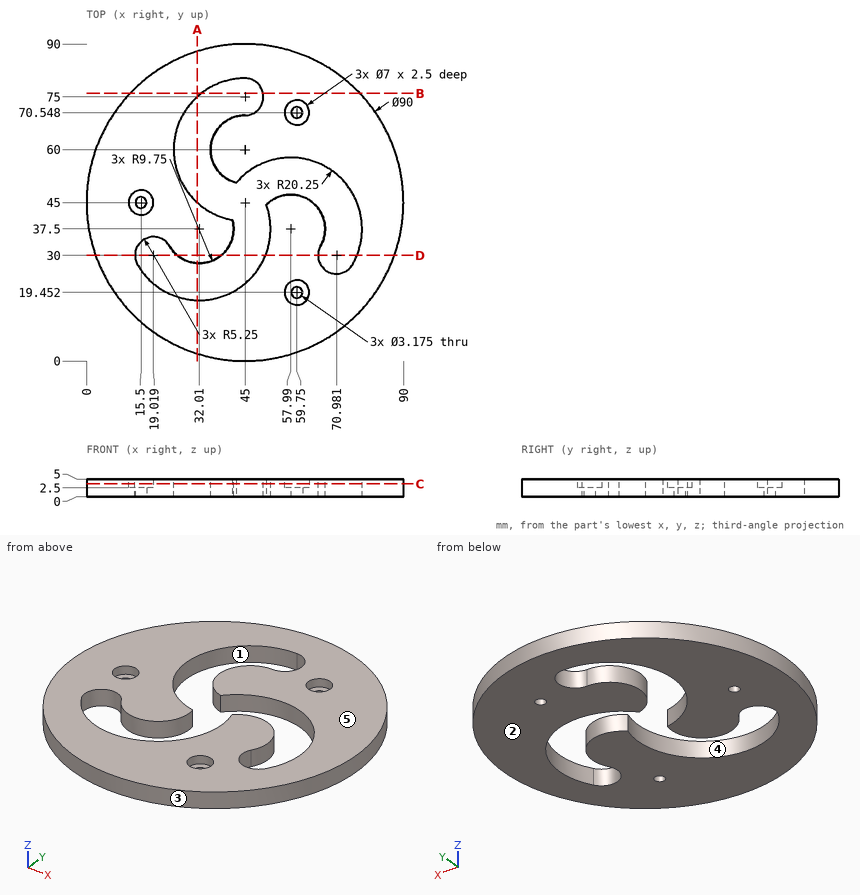
Here's the drawing with two shaded views (mm, measured from the low corner). I have some questions. A direction names the side the tool comes from. Round coordinates to 2 decimals unless told otherwise and drop trailing zeros. Loops run counter-clockwise (first coordinate to the right, second up) from the corner with the lowest first, then second, coordinate; pieces in that order, holes last. Notation, with made-up numbers: M 39,-40 L 74,-40 A33 ccw 74,-10 Z; hole C 41,-34 d1. An arc over 180 degrees is marked long. Answer as CSV lines item,"result".
1) Imagine slicing it at B-B on y = 76. List the corners of the cut face in (x, z) for me.
From the geometry:
outline,"M 12.38,0 L 32.59,0 L 32.59,5 L 12.38,5 Z; M 50.15,0 L 77.62,0 L 77.62,5 L 50.15,5 Z"
2) We'd pull the mould along X, two halves only. Please class the marked faces 3, 4 and 5: released by +X, released by -X, zero draft, split by the parting line, or undercut.
From the geometry:
face 3,"split by the parting line"
face 4,"undercut"
face 5,"zero draft"
3) Which directions (+Z, -Z, +X, -X, +Y, -Y) give clear straight access to the entire face, cutting with the end or side of a thin tool? Please do the marked faces 1 and 2.
From the geometry:
face 1,"+Z, -Z"
face 2,"-Z, +X, -X, +Y, -Y"
4) For pin 1 Ø3.5 at (x, y) = (59.75, 70.55) entering from +Z; pin 2 Ø3 at (x, z) = (57, 3) entering from -Y; pin 3 Ø1 at (y, z) = (10.5, 3) entering from +X, each with a flat end and sliding along its axis, tell me the tip position at first contact or that it passes through.
From the geometry:
pin 1,"z = 2.5"
pin 2,"y = 1.24"
pin 3,"x = 74.48"
5) If I drill on probe 1 along Y at (x, z) = (15.5, 3.5) (1 decimal); probe 2 along X at (y, z) = (31, 0.55) (1 decimal); probe 3 along Y at (x, z) = (59.75, 1) (1 decimal), over which ranges is the centre line in solid material (lowest first)?
From the geometry:
probe 1,"11 to 25.8, 33.9 to 41.5, 48.5 to 79"
probe 2,"2.2 to 13.9, 24.7 to 39.3, 51.2 to 65.8, 77.2 to 87.8"
probe 3,"2.5 to 17.9, 21 to 47.1, 57.7 to 69, 72.1 to 87.5"
6) Imagine slicing it at A-A on x = 31.5. List the corners of the cut face in (y, z) for me, and give its area (3 significant figures).
From the geometry:
outline,"M 2.07,0 L 17.26,0 L 17.26,5 L 2.07,5 Z; M 27.76,0 L 44.91,0 L 44.91,5 L 27.76,5 Z; M 75.09,0 L 87.93,0 L 87.93,5 L 75.09,5 Z"
area,"226 mm^2"
7) Imagine slicing it at C-C on z = 3.65. Count the separate pieces of the cut face and the enclosed holes in it, and give its area (3 significant figures).
From the geometry:
separate pieces,"1"
enclosed holes,"4"
area,"4,680 mm^2"
8) Imagine slicing it at D-D on y = 30. List the corners of the cut face in (x, z) for me.
From the geometry:
outline,"M 2.57,0 L 13.77,0 L 13.77,5 L 2.57,5 Z; M 25.78,0 L 38.24,0 L 38.24,5 L 25.78,5 Z; M 50.82,0 L 65.73,0 L 65.73,5 L 50.82,5 Z; M 76.8,0 L 87.43,0 L 87.43,5 L 76.8,5 Z"
